Source: CAD feature listing. Evaluate the final solid. Frame: model axes, mm. A direction names the side the tool comes from. Round coordinates to 2 decimals unless told otherwise and drop trailing zeros. Order: outer loops, then holes, each group sorted by start corner. A loop starts at its lowest first (then second) coordinate and runs counter-clockwise, first axis right, second up.
```python
from build123d import *

# Parameters (mm, degrees)
F0_R     = 6.35
F0_R_2   = 3.175
F1_DEPTH = 3.175
F2_R     = 11.1125
F2_R_2   = 3.175
F3_DEPTH = 14.478
F4_R     = 8.001
F5_DEPTH = 12.7


with BuildPart() as f1:
    # F0 (on Top) → F1 (new body)
    with BuildSketch(Plane.XY):
        Circle(F0_R)
        Circle(F0_R_2, mode=Mode.SUBTRACT)
    extrude(amount=F1_DEPTH)

    # F2 (on face) → F3 (join)
    with BuildSketch(Plane.XY.offset(3.175)):
        Circle(F2_R)
        Circle(F2_R_2, mode=Mode.SUBTRACT)
    extrude(amount=F3_DEPTH)

    # F4 (on face) → F5 (cut)
    with BuildSketch(Plane.XY.offset(17.653)):
        Circle(F4_R)
    extrude(amount=-F5_DEPTH, mode=Mode.SUBTRACT)


solid = f1.part
```
1. Access query for faces 4 (the face through (-2, 3, 0)), 5 (the face through (5, -5, 3.175)), 6 (the face through (3.4, 0.1, 4.953)). Directions: +Z, -Z, +X, -X, +Y, -Y. A direction counts if a zero-diameter tool reaches every point of the face in a straight line with its end or side. Return the directions, or none.
2. Section C-C on y = -5.5. Return loops of the section in (x, z) (3 decimals).
3. Section D-D on x = -4.5. Return loops of the section in (y, z) (3 decimals).
4. Pull-direction query (X, two-part tool) for faces 1 (the face through (-1.38, -6.2, 1.57)), 2 (the face through (-1.73, -7.81, 11.39)), 3 (the face through (-8, 3, 17.653)); classes: released by +X, released by -X, zero draft, split by the parting line, or undercut.
5. First-contact query: pin 1 (8 mm diameter, centred on x = 8, z = 4, fed in from +Y); pin 2 (1.5 mm diameter, centred on y = 3, z = 9, fed in from -X); pin 3 (8 mm diameter, centred on y = -7.5, z = 11, fed in from -X); pin 4 (4 mm diameter, centred on x = 0, y = 0, fed in from +Z). Flat tips, straight axial feed; report the tip coordinate or a pass-through.
6. Line query: line 1 along Y through (x, z) = (0, 2.35) (3 decimals); line 2 along Y through (x, z) = (0, 9.25); line 3 along Z through (x, y) = (1.25, 9.75) (3 decimals). Output: solid intervals per line, ascending.
Result:
1. face 4: -Z, +X, -X, +Y, -Y
1. face 5: -Z
1. face 6: +Z
2. outline: (-9.656, 3.175) - (-3.174, 3.175) - (-3.174, 0) - (3.174, 0) - (3.174, 3.175) - (9.656, 3.175) - (9.656, 17.653) - (5.811, 17.653) - (5.811, 4.953) - (-5.811, 4.953) - (-5.811, 17.653) - (-9.656, 17.653) - close
3. outline: (-10.161, 3.175) - (-4.48, 3.175) - (-4.48, 0) - (4.48, 0) - (4.48, 3.175) - (10.161, 3.175) - (10.161, 17.653) - (6.616, 17.653) - (6.616, 4.953) - (-6.616, 4.953) - (-6.616, 17.653) - (-10.161, 17.653) - close
4. face 1: split by the parting line
4. face 2: undercut
4. face 3: zero draft
5. pin 1: stops at y = 10.37
5. pin 2: stops at x = -10.88
5. pin 3: stops at x = -10.55
5. pin 4: passes through
6. line 1: y = -6.35 to -3.175, 3.175 to 6.35
6. line 2: y = -11.11 to -8, 8 to 11.11
6. line 3: z = 3.175 to 17.653
